```python
from build123d import *

# Parameters (mm, degrees)
SKETCH1_W           = 300
SKETCH1_H           = 300
SKETCH1_W_2         = 100
SKETCH1_H_2         = 100
BOSS_EXTRUDE1_DEPTH = 15
FILLET1_R           = 50


with BuildPart() as part:
    # Sketch1 → Boss-Extrude1 (new body)
    with BuildSketch(Plane(origin=(0, 0, 0), x_dir=(1, 0, 0), z_dir=(0, 1, 0))):
        with Locations((150, 150)):
            Rectangle(SKETCH1_W, SKETCH1_H)
        with Locations((50, -50)):
            Rectangle(SKETCH1_W_2, SKETCH1_H_2)
    extrude(amount=BOSS_EXTRUDE1_DEPTH)

    # Fillet1
    fillet1_edges = [part.edges().sort_by_distance(p)[0] for p in [
        (0, 7.5, -300),
        (0, 7.5, 100),
        (300, 7.5, -300),
        (300, 7.5, 0),
        (100, 7.5, 100),
        (100, 7.5, 0),
    ]]
    fillet(fillet1_edges, radius=FILLET1_R - 0.0001)  # a hair under: the kernel refuses the full size


solid = part.part
```
Read the model definition and answer for the solid it produces. Units are mm, in the model's axes. A direction names the side the tool comes from. Round coordinates to 2 decimals unless told otherwise and drop trailing zeros. Loops run counter-clockwise (first coordinate to the right, second up) from the corner with the lowest first, then second, coordinate; pieces in that order, holes last. Notation, with made-up numbers: (-38.5, 0.5) -> (-19.5, 0.5) arc R16 ccw to (-19.5, 27.5) -> close; hole circle Ø4 at (18.25, -15.5). An arc over 180 degrees is marked (long way). One line per item, written item: value.
1) The mould has two halves that part along Y. Classify faces 1 (the face through (148, 0, -147)), 2 (the face through (148, 15, -147)), 3 (the face through (149, 7, -300)): pulls with the +Y half, pulls with the -Y half, needs draft (parallel to the pull), parting line crosses it, or undercut.
Answer list:
face 1: pulls with the -Y half
face 2: pulls with the +Y half
face 3: needs draft
2) Flat-ended cylindrical pins translate along their axes: P1, Ø2, axis at y = 10.5, z = 18.5, coming from the +X side; P2, Ø1.5, axis at y = 10.5, z = -256, coming from the -X side. Find the tip coordinate at first contact, or state that the pin passes through.
Answer list:
P1: stops at x = 112
P2: stops at x = 0.28
3) Consider L1, parallel to Z at x = 171, y = 7.75; L2, parallel to Z at x = 70, y = 13.5; L3, parallel to X at y = 10.25, z = -34. Determine where each line is inside the solid, lowest interval first. Write a range as [from, to].
Answer list:
L1: z = [-300, 0]
L2: z = [-300, 95.83]
L3: x = [0, 297.37]
4) A cutting plane is placed at B-B (x = 166). Determine the outline of the cut face in (y, z), and give its area (3 significant figures).
Answer list:
outline: (0, -300) -> (15, -300) -> (15, 0) -> (0, 0) -> close
area: 4,500 mm²
5) For faces 4 (the face through (199, 7, 0)), 5 (the face through (0, 7, -102)), determine the directions among +Z, -Z, +X, -X, +Y, -Y from which every point of the face is accessible in a straight line to the end or side of a thin tool.
Answer list:
face 4: +Z, +X, +Y, -Y
face 5: +Z, -Z, -X, +Y, -Y
6) A cutting plane is placed at C-C (z = 4.5). Determine the outline of the cut face in (x, y).
Answer list:
outline: (0, 0) -> (129.27, 0) -> (129.27, 15) -> (0, 15) -> close
